Here's how the part is built. I have some questions about the finished solid (model axes, mm). A direction names the side the tool comes from. Coordinates: 2 decimals unless noted, no trailing zeros. Write each loop counter-clockwise with the first axis right and the second up, starting at its lowest first coordinate (ties: lowest second). Pieces come first, ordered by that corner, then holes.
```python
from build123d import *

# Parameters (mm, degrees)
SKETCH2_W           = 25
SKETCH2_H           = 12
SKETCH2_R           = 1.75
SKETCH2_R_2         = 2.1
BOSS_EXTRUDE1_DEPTH = 18
SKETCH7_W           = 7
SKETCH7_H           = 4
CUT_EXTRUDE3_DEPTH  = 10
SKETCH9_W           = 5.5
SKETCH9_H           = 3
CUT_EXTRUDE4_DEPTH  = 8
FILLET1_R           = 1
CHAMFER1_SIZE       = 1


with BuildPart() as part:
    # Sketch2 → Boss-Extrude1 (new body)
    with BuildSketch(Plane(origin=(0, 0, 0), x_dir=(1, 0, 0), z_dir=(0, 1, 0))):
        Rectangle(SKETCH2_W, SKETCH2_H)
        with Locations(Location((-7.5, 0, 0), (0, 0, 270))):
            Circle(SKETCH2_R, mode=Mode.SUBTRACT)
        with Locations(Location((7.5, 0, 0), (0, 0, 270))):
            Circle(SKETCH2_R_2, mode=Mode.SUBTRACT)
    extrude(amount=BOSS_EXTRUDE1_DEPTH)

    # Sketch7 → Cut-Extrude3 (cut)
    with BuildSketch(Plane(origin=(12.5, 0, 0), x_dir=(0, 0, -1), z_dir=(1, 0, 0))):
        with Locations((0, 5)):
            Rectangle(SKETCH7_W, SKETCH7_H)
    extrude(amount=-CUT_EXTRUDE3_DEPTH, mode=Mode.SUBTRACT)

    # Sketch9 → Cut-Extrude4 (cut)
    with BuildSketch(Plane.ZY.offset(12.5)):
        with Locations((0, 4.5)):
            Rectangle(SKETCH9_W, SKETCH9_H)
    extrude(amount=-CUT_EXTRUDE4_DEPTH, mode=Mode.SUBTRACT)

    # Fillet1
    fillet1_edges = [part.edges().sort_by_distance(p)[0] for p in [
        (12.5, 9, 6),
        (-12.5, 9, 6),
        (-12.5, 9, -6),
        (12.5, 9, -6),
    ]]
    fillet(fillet1_edges, radius=FILLET1_R)

    # Chamfer1
    chamfer1_edges = [part.edges().sort_by_distance(p)[0] for p in [
        (0, 0, 6),
        (0, 18, 6),
        (12.5, 0, 0),
        (-12.5, 0, 0),
        (0, 0, -6),
        (12.207106781, 0, 5.707106781),
        (12.207106781, 0, -5.707106781),
        (-12.207106781, 0, -5.707106781),
        (-12.207106781, 0, 5.707106781),
        (-12.5, 18, 0),
        (12.5, 18, 0),
        (0, 18, -6),
        (12.207106781, 18, 5.707106781),
        (12.207106781, 18, -5.707106781),
        (-12.207106781, 18, -5.707106781),
        (-12.207106781, 18, 5.707106781),
    ]]
    chamfer(chamfer1_edges, length=CHAMFER1_SIZE)


solid = part.part
```
1) On a 3-axis mill with a long thin cutter (end or side, diameter ignored), from which of +Z, -Z, +X, -X, +Y, -Y can I reach the whole of each face in a straight line? I mean faces 1 (the face through (-0.2, 17.5, 5.5)), 2 (the face through (-9.4, 3, 0)), 3 (the face through (8, 5, 3.5)). Say none if no direction works.
Values follow:
face 1: +Z, +X, -X, +Y
face 2: -X
face 3: +X
2) I need wall thicknesses on probe 1 along X at (y, z) = (2.2, 0); probe 2 along Z at (x, y) = (7.5, 10.5); probe 3 along Z at (x, y) = (4.5, 3.5). Which ranges of each line are inside material? Lowest first, please.
Values follow:
probe 1: x = -12.5 to -9.25, -5.75 to 5.4, 9.6 to 12.5
probe 2: z = -6 to -2.1, 2.1 to 6
probe 3: z = -6 to -3.5, 3.5 to 6
3) Imagine slicing it at C-C on y = 5.5. Please give me the cut outline in (x, z).
Values follow:
outline: (-12.5, -5) arc R1 ccw to (-11.5, -6) - (11.5, -6) arc R1 ccw to (12.5, -5) - (12.5, -3.5) - (2.5, -3.5) - (2.5, 3.5) - (12.5, 3.5) - (12.5, 5) arc R1 ccw to (11.5, 6) - (-11.5, 6) arc R1 ccw to (-12.5, 5) - (-12.5, 2.75) - (-4.5, 2.75) - (-4.5, -2.75) - (-12.5, -2.75) - close
4) Imagine slicing it at B-B on z = 0. Count the separate pieces of the cut face and the enclosed holes in it, then the cut area to 3 significant figures.
Values follow:
separate pieces: 5
enclosed holes: 0
area: 273 mm2
5) Imagine slicing it at A-A on x = -7.5. Please give me the cut outline in (y, z), then the cut area to 3 significant figures.
Values follow:
outline: (0, -5) - (1, -6) - (17, -6) - (18, -5) - (18, -1.75) - (6, -1.75) - (6, -2.75) - (3, -2.75) - (3, -1.75) - (0, -1.75) - close; (0, 1.75) - (3, 1.75) - (3, 2.75) - (6, 2.75) - (6, 1.75) - (18, 1.75) - (18, 5) - (17, 6) - (1, 6) - (0, 5) - close
area: 145 mm2
6) Imagine slicing it at D-D on y = 9. Please give me the cut outline in (x, z), then the cut area to 3 significant figures.
Values follow:
outline: (-12.5, -5) arc R1 ccw to (-11.5, -6) - (11.5, -6) arc R1 ccw to (12.5, -5) - (12.5, 5) arc R1 ccw to (11.5, 6) - (-11.5, 6) arc R1 ccw to (-12.5, 5) - close; hole circle Ø3.5 at (-7.5, 0); hole circle Ø4.2 at (7.5, 0)
area: 276 mm2
7) We'd pull the mould along Y, two halves only. Please class faces 4 (the face through (-12, 0.5, -0.1)), 5 (the face through (-12, 17.5, -0.1)), 6 (the face through (8, 5, -3.5)), 7 (the face through (-9.4, 6, 0)): pulls with the +Y half, pulls with the -Y half, needs draft (parallel to the pull), parting line crosses it, or undercut.
Values follow:
face 4: pulls with the -Y half
face 5: pulls with the +Y half
face 6: undercut
face 7: undercut
